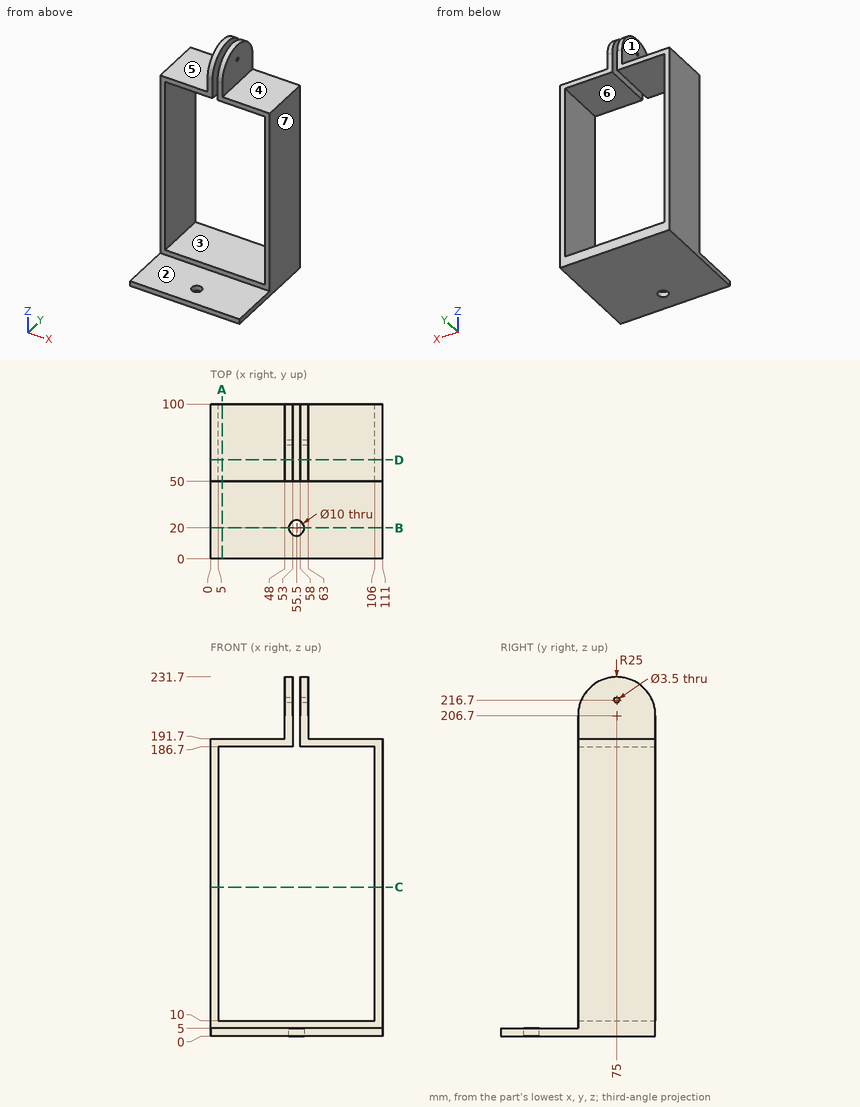
Job drawing, mm, ordinate dimensions from the low corner. One solid piece. A direction names the side the tool comes from. Coordinates: 2 decimals unless noted, no trailing zeros. Write each loop counter-clockwise with the first axis right and the second up, starting at its lowest first coordinate (ties: lowest second). Pieces come first, ordered by that corner, then holes.
Item 1: Slice it at A-A (x = 7.5). Write the cut outline in (y, z), and give its area (3 significant figures).
Item 2: Slice it at C-C (z = 96). Write the cut outline in (x, y), and give its area (3 significant figures).
Item 3: Probe line 1 (Z direction, x = 49.65, y = 75); line 2 (X direction, y = 63, z = 20); line 3 (Y direction, x = 55.5, z = 2.8). List the from-to ranges inside material, lowest first.
Item 4: Slice it at B-B (y = 20). Write the cut outline in (x, z).
Item 5: Pin check, flat tips, straight feed: pin 1 (15 mm diameter, centred on x = 40.5, y = 31.5, fed in from +Z); pin 2 (4 mm diameter, centred on y = 75, z = 216.7, fed in from -X); pin 3 (15 mm diameter, centred on x = 50.5, y = 67.5, fed in from +Z). Stop position of each tip, or through.
Item 6: Slice it at D-D (y = 64). Write the cut outline in (x, z).
Item 7: Mould opens along Z. For the marked faces 5, 6 and 7 say: released by +Z, released by -Z, zero draft, split by the parting line, or undercut.
Item 8: Which spindle directions (+Z, -Z, +X, -X, +Y, -Y) get a long thin tool onto all of the face, cutting with end or side? Do the marked faces 1, 2, 3 and 4. Say none if no direction does.
Results found:
1. outline: (0, 0) - (100, 0) - (100, 10) - (50, 10) - (50, 5) - (0, 5) - close; (50, 186.7) - (100, 186.7) - (100, 191.7) - (50, 191.7) - close
1. area: 1,000 mm2
2. outline: (0, 50) - (5, 50) - (5, 100) - (0, 100) - close; (106, 50) - (111, 50) - (111, 100) - (106, 100) - close
2. area: 500 mm2
3. line 1: z = 0 to 10, 186.7 to 214.95, 218.45 to 231.7
3. line 2: x = 0 to 5, 106 to 111
3. line 3: y = 0 to 15, 25 to 100
4. outline: (0, 0) - (50.5, 0) - (50.5, 5) - (0, 5) - close; (60.5, 0) - (111, 0) - (111, 5) - (60.5, 5) - close
5. pin 1: stops at z = 5
5. pin 2: stops at x = 48
5. pin 3: stops at z = 231.7
6. outline: (0, 0) - (111, 0) - (111, 191.7) - (63, 191.7) - (63, 229.15) - (58, 229.15) - (58, 186.7) - (106, 186.7) - (106, 10) - (5, 10) - (5, 186.7) - (53, 186.7) - (53, 229.15) - (48, 229.15) - (48, 191.7) - (0, 191.7) - close
7. face 5: released by +Z
7. face 6: undercut
7. face 7: zero draft
8. face 1: +Z, -X, +Y, -Y
8. face 2: +Z, +X, -X, -Y
8. face 3: +Y, -Y
8. face 4: +Z, +X, +Y, -Y
